Print and shaded views of the part. All mm, measured from the part's lowest x, y and z. A direction names the side the tool comes from. Round coordinates to 2 decimals unless told otherwise and drop trailing zeros. Order: outer loops, then holes, each group sorted by start corner. A loop starts at its lowest first (then second) coordinate and runs counter-clockwise, first axis right, second up. Notation, with made-up numbers: M 87.25,82.5 L 128.25,82.5 A26 ccw 128.25,105.5 Z; hole C 68,6 d11. An arc over 180 degrees is marked long. Use CSV: the item, a comma, the result in double quotes.
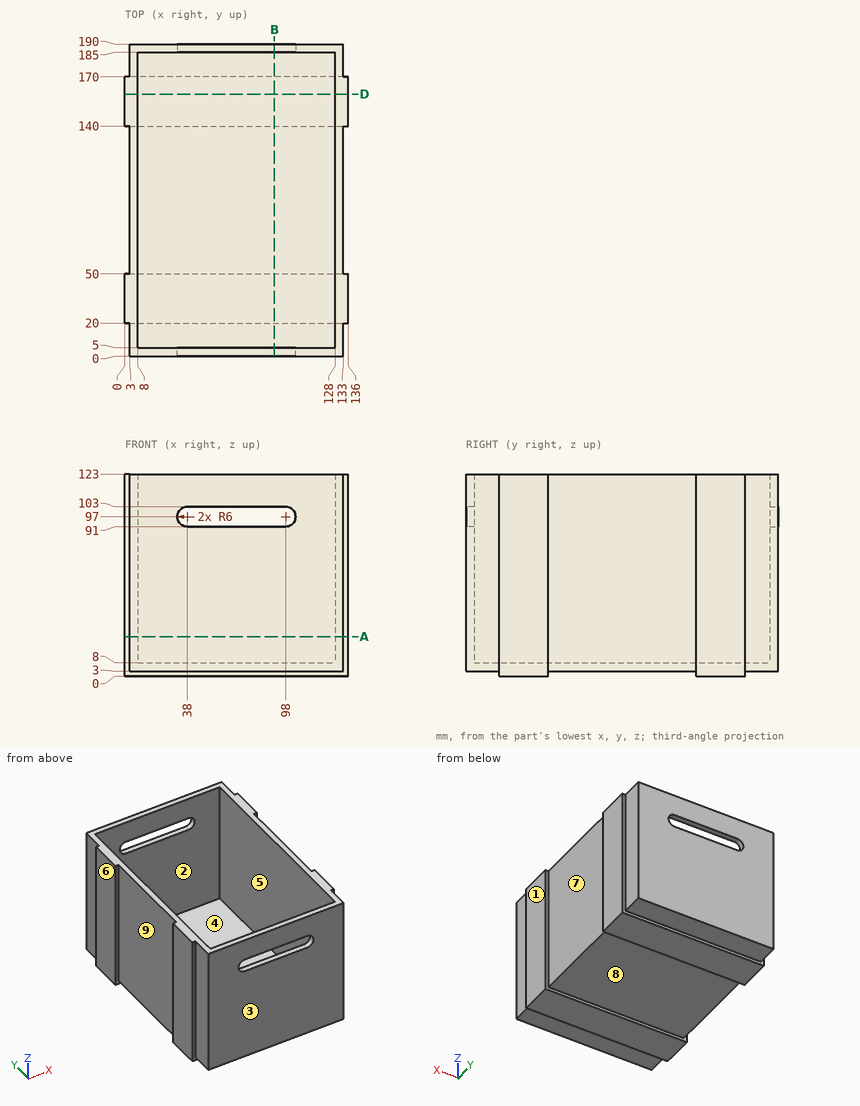
(1) Cut at D-D, the plane y = 159.5. Give the cut face in (x, z), and give its area (3 significant figures).
Answer block:
outline,"M 0,0 L 136,0 L 136,123 L 128,123 L 128,8 L 8,8 L 8,123 L 0,123 Z"
area,"2,930 mm²"
(2) Cut at B-B, the plane x = 91. Give the cut face in (y, z).
Answer block:
outline,"M 0,3 L 20,3 L 20,0 L 50,0 L 50,3 L 140,3 L 140,0 L 170,0 L 170,3 L 190,3 L 190,91 L 185,91 L 185,8 L 5,8 L 5,91 L 0,91 Z; M 0,103 L 5,103 L 5,123 L 0,123 Z; M 185,103 L 190,103 L 190,123 L 185,123 Z"
(3) Wall check: line 1 (X direction, y = 105, z = 17.5); line 2 (Y direction, x = 12.5, z = 34.5); line 3 (X direction, y = 141, z = 51). Give the ranges that are in metal, low to high. Write a range as from..to.
Answer block:
line 1,"x = 3..8, 128..133"
line 2,"y = 0..5, 185..190"
line 3,"x = 0..8, 128..136"
(4) Cut at A-A, the plane z = 24. Give the cut face in (x, y), and give its area (3 significant figures).
Answer block:
outline,"M 0,20 L 3,20 L 3,0 L 133,0 L 133,20 L 136,20 L 136,50 L 133,50 L 133,140 L 136,140 L 136,170 L 133,170 L 133,190 L 3,190 L 3,170 L 0,170 L 0,140 L 3,140 L 3,50 L 0,50 Z; hole M 8,5 L 128,5 L 128,185 L 8,185 Z"
area,"3,460 mm²"
(5) Two-plate mould, pull along Y, no slides. Class the marked faces 1, 2, 3 and 4: released by +Y, released by -Y, zero draft, split by the parting line, or undercut.
Answer block:
face 1,"zero draft"
face 2,"undercut"
face 3,"released by -Y"
face 4,"undercut"
(6) Drop flat-ended pins along their axis: pin 1 (6 mm diameter, centred on y = 182.5, z = 81, fed in from +X); pin 2 (5.5 mm diameter, centred on x = 60, y = 186.5, fed in from -Z); pin 3 (6 mm diameter, centred on y = 8.5, z = 89.5, fed in from -X); pin 4 (6 mm diameter, centred on x = 81.5, z = 28.5, fed in from -Y). Give the stop position or say it passes through.
Answer block:
pin 1,"stops at x = 133"
pin 2,"stops at z = 3"
pin 3,"stops at x = 3"
pin 4,"stops at y = 0"
(7) Tool access for the marked faces 5, 6, 7, 8 and 9: list every direction of +Z, -Z, +X, -X, +Y, -Y with a clear straight run to the whole face (end or side of a thin tool).
Answer block:
face 5,"+Z"
face 6,"+Z, -Z, -X, +Y, -Y"
face 7,"+Z, -Z, +X"
face 8,"-Z, +X, -X"
face 9,"+Z, -Z, -X"
